Input: part model. Units: mm. Frame: model coordinates. Coordinates: 2 decimals unless noted, no trailing zeros. Loops run counter-clockwise (first coordinate to the right, second up) from the corner with the lowest first, then second, coordinate; pieces in that order, holes last. Notation, with made-up numbers: (39, 22.5) -> (89, 22.5) arc R5 ccw to (89, 27.5) -> close; hole circle Ø7 at (55, 79.25). An arc over 180 degrees is marked (long way). Put each result on its own line as item: value. Start each with the question number.
1) Cut plane A-A (z = -0.7). Return the cut outline in (x, y).
2) Cut plane C-C (y = 37). Return the cut outline in (x, z).
3) Material intervals for L1, parallel to Y at x = -3, z = 0.5; L2, parallel to X at y = -6.5, z = -1.1; L3, parallel to Y at x = -14, z = 1.8, sorted ascending.
4) Contact query for flat-ended pins moving along their axis: P1, Ø1.5, axis at y = 46.5, z = -1.5, coming from the -X side; P2, Ø2, axis at x = -30, z = 0, coming from the +Y side; P3, Ø2, axis at x = -9, z = 0.5, coming from the -Y side. Output: stop coordinate, or through.
5) Cut plane D-D (x = -24.5). Return the cut outline in (y, z), plus the area to 3 significant figures.
6) Cut plane B-B (y = -2). Return the cut outline in (x, z), plus the area to 3 significant figures.
from build123d import *

# Parameters (mm, degrees)
PAD_DEPTH    = 2
SKETCH_W     = 10
SKETCH_H     = 6
POCKET_DEPTH = 4.001


with BuildPart() as part:
    # CopySketch004 → Pad (new body, symmetric)
    with BuildSketch(Plane.XY):
        with BuildLine():
            Line((-36.508492, 11.060009), (-1.723702, 11.060009))
            ThreePointArc((-1.723702, 11.060009), (7.733856, 14.212769), (13.407871, 22.409771))
            Line((13.407871, 22.409771), (24.319128, 59.832547))
            Line((24.319128, 59.832547), (51.226102, 59.832547))
            Line((51.226102, 59.832547), (51.226102, -16.067453))
            Line((24.319128, -16.067453), (51.226102, -16.067453))
            Line((23.401691, -4.060687), (24.319128, -16.067453))
            ThreePointArc((23.401691, -4.060687), (22.843077, -1.909417), (21.705474, 0))
            Line((16, 0), (21.705474, 0))
            Line((16, -10), (16, 0))
            Line((-16, -10), (16, -10))
            Line((-16, -10), (-36.508492, -0.144815))
            Line((-36.508492, 2.549264), (-36.508492, -0.144815))
            Line((-26.508492, 2.549264), (-36.508492, 2.549264))
            Line((-26.508492, 6.549264), (-26.508492, 2.549264))
            Line((-36.508492, 6.549264), (-26.508492, 6.549264))
            Line((-36.508492, 11.060009), (-36.508492, 6.549264))
        make_face()
    extrude(amount=PAD_DEPTH, both=True)

    # Sketch (on Face19 of Pad) → Pocket (cut, through all)
    with BuildSketch(Plane.XY.offset(2)):
        with Locations((0, -7)):
            Rectangle(SKETCH_W, SKETCH_H)
    extrude(amount=-POCKET_DEPTH, mode=Mode.SUBTRACT)


solid = part.part
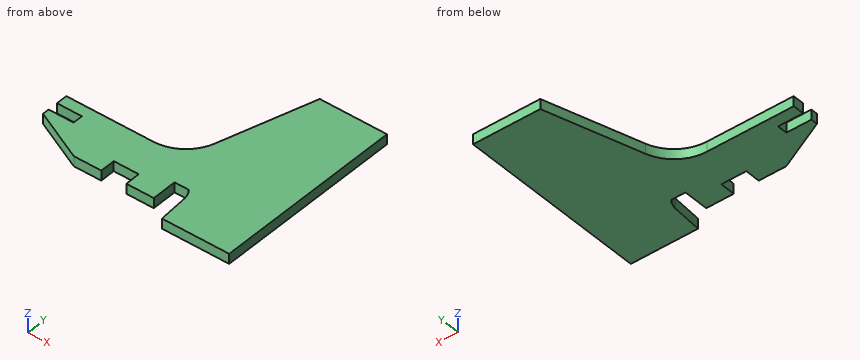
Results found:
1. outline: (-36.51, -0.14) -> (-16, -10) -> (-5, -10) -> (-5, -4) -> (5, -4) -> (5, -10) -> (16, -10) -> (16, 0) -> (21.71, 0) arc R7.87 cw to (23.4, -4.06) -> (24.32, -16.07) -> (51.23, -16.07) -> (51.23, 59.83) -> (24.32, 59.83) -> (13.41, 22.41) arc R15.76 cw to (-1.72, 11.06) -> (-36.51, 11.06) -> (-36.51, 6.55) -> (-26.51, 6.55) -> (-26.51, 2.55) -> (-36.51, 2.55) -> close
2. outline: (17.66, -2) -> (51.23, -2) -> (51.23, 2) -> (17.66, 2) -> close
3. L1: y = -4 to 11.06
3. L2: x = -23.28 to -5, 5 to 16, 23.59 to 51.23
3. L3: y = -10 to 11.06
4. P1: stops at x = 20.21
4. P2: stops at y = 11.06
4. P3: stops at y = -10
5. outline: (-5.92, -2) -> (11.06, -2) -> (11.06, 2) -> (-5.92, 2) -> close
5. area: 67.9 mm2
6. outline: (-32.65, -2) -> (16, -2) -> (16, 2) -> (-32.65, 2) -> close; (22.88, -2) -> (51.23, -2) -> (51.23, 2) -> (22.88, 2) -> close
6. area: 308 mm2
